Here's how the part is built. I have some questions about the finished solid (model axes, mm). Face numbers are marked on the shaded views. A direction names the side the tool comes from. Give positions to 0.01 mm unless a question says otherwise; leave off trailing zeros. Write each loop counter-clockwise with the first axis right and the second up, starting at its lowest first coordinate (ties: lowest second). Pieces come first, ordered by that corner, then holes. Notation, with made-up numbers: M 52.5,-36.75 L 100.5,-36.75 A25 ccw 100.5,-11.75 Z; hole C -16.75,84.25 d4. An arc over 180 degrees is marked long. Answer as CSV lines item,"result". Start each with the question number.
Q1. Suppose I cut it at A-A (x = 0). Write out the boundary of the cut face in (y, z), then the cut area to 3 significant figures.
Q2. If I drill on line 1 along Z through (x, y) = (0, 0.15); line 2 along Z through (x, y) = (0, 3); line 3 along Y through (x, z) = (-1.75, -12.25), over which ranges is the centre line in solid material (lowest first)?
Q3. Suppose I cut it at D-D (x = -8). Write out the boundary of the cut face in (y, z), then the cut area to 3 significant figures.
Q4. Thinking about a two-plate mould opening in X: for the marked faces 1 and 2, which applies, +X half, -X half, draft (parallel to the pull), parting line (faces both ways), or undercut?
Q5. On a 3-axis mill with a long thin cutter (end or side, diameter ignored), from which of +Z, -Z, +X, -X, +Y, -Y can I reach the whole of each face in a straight line? I mean the marked faces 3 and 4. Say none if no direction works.
Q6. Suppose I cut it at B-B (z = 0). Write out the boundary of the cut face in (x, y).
Q7. For pin 1 (9.5 mm diameter, centred on x = 0, z = 0, fed in from +Y); pin 2 (1.5 mm diameter, centred on x = -3, y = 6, fed in from -Z); pin 3 (2 mm diameter, centred on y = 4, z = -3.5, fed in from -X) (3 decimals); pin 4 (3 mm diameter, centred on x = -7.5, y = 6, fed in from +Z), each with a flat end and sliding along its axis, tell me the tip position at first contact or that it passes through.
Q8. Suppose I cut it at C-C (y = 5.75). Write out the boundary of the cut face in (x, z), then the cut area to 3 significant figures.
Autodesk Inventor part; units mm, degrees
ref_plane "YZ Plane" through (0, 0, 0) normal (1, 0, 0) x (0, 1, 0)
ref_plane "XZ Plane" through (0, 0, 0) normal (0, 1, 0) x (-1, 0, 0)
ref_plane "XY Plane" through (0, 0, 0) normal (0, 0, 1) x (1, 0, 0)
sketch "スケッチ1" plane through (0, 0, 0) normal (0, 1, 0) x (-1, 0, 0)
  circle A0 centre (0, 0) radius 6
  circle A1 centre (0, 0) radius 14
  dimension "d0" = 12
  dimension "d1" = 28
extrude "押し出し1" add sketch "スケッチ1" along normal blind 8
sketch "スケッチ2" plane through (0, 0, 0) normal (0, -1, 0) x (1, 0, 0)
  circle A0 centre (0, 0) radius 7.5
  circle A1 centre (0, 0) radius 13
  dimension "d4" = 15
  dimension "d5" = 26
extrude "押し出し2" cut sketch "スケッチ2" against normal blind 0.2
sketch "スケッチ3" plane through (0, 8, 0) normal (0, 1, 0) x (1, 0, 0)
  circle A0 centre (0, 0) radius 7.5
  circle A1 centre (0, 0) radius 13
  dimension "d8" = 15
  dimension "d9" = 26
extrude "押し出し3" cut sketch "スケッチ3" against normal blind 0.2
properties part number "Bearing_6001Z" material "ステンレス鋼"
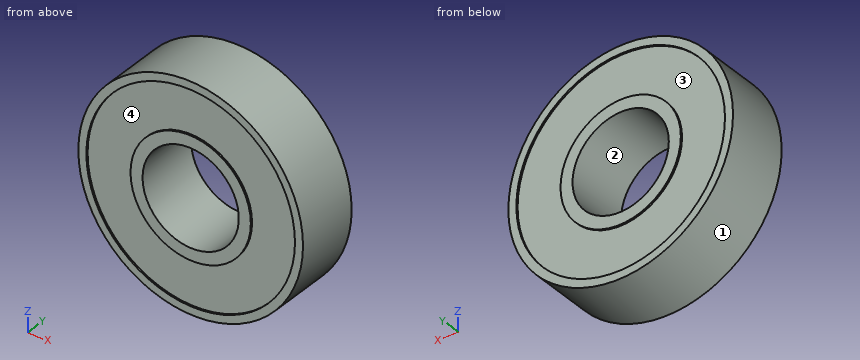
Resolved:
1,outline,"M 0,-14 L 8,-14 L 8,-13 L 7.8,-13 L 7.8,-7.5 L 8,-7.5 L 8,-6 L 0,-6 L 0,-7.5 L 0.2,-7.5 L 0.2,-13 L 0,-13 Z; M 0,6 L 8,6 L 8,7.5 L 7.8,7.5 L 7.8,13 L 8,13 L 8,14 L 0,14 L 0,13 L 0.2,13 L 0.2,7.5 L 0,7.5 Z"
1,area,"124 mm^2"
2,line 1,"-14 to -13, -7.5 to -6, 6 to 7.5, 13 to 14"
2,line 2,"-14 to -6, 6 to 14"
2,line 3,"0.2 to 7.8"
3,outline,"M 0,-11.49 L 8,-11.49 L 8,-10.25 L 7.8,-10.25 L 7.8,10.25 L 8,10.25 L 8,11.49 L 0,11.49 L 0,10.25 L 0.2,10.25 L 0.2,-10.25 L 0,-10.25 Z"
3,area,"176 mm^2"
4,face 1,"parting line"
4,face 2,"undercut"
5,face 3,"+Y"
5,face 4,"-Y"
6,outline,"M -14,0 L -13,0 L -13,0.2 L -7.5,0.2 L -7.5,0 L -6,0 L -6,8 L -7.5,8 L -7.5,7.8 L -13,7.8 L -13,8 L -14,8 Z; M 6,0 L 7.5,0 L 7.5,0.2 L 13,0.2 L 13,0 L 14,0 L 14,8 L 13,8 L 13,7.8 L 7.5,7.8 L 7.5,8 L 6,8 Z"
7,pin 1,"through"
7,pin 2,"z = -13.82"
7,pin 3,"x = -13.775"
7,pin 4,"z = 12.65"
8,outline,"C 0,0 d28; hole C 0,0 d12"
8,area,"503 mm^2"
